Source: CAD feature listing. Evaluate the final solid. Frame: model axes, mm. Face numbers are marked on the shaded views. Give positions to 0.01 mm unless a question says otherwise; leave off trailing zeros. Loops run counter-clockwise (first coordinate to the right, second up) from the corner with the lowest first, then second, coordinate; pieces in that order, holes last. Notation, with made-up numbers: M -1.5,22 L 5.5,22 A13 ccw 5.5,31 Z; hole C 12,-29.5 d10. An arc over 180 degrees is marked long. Write item = value, one per line.
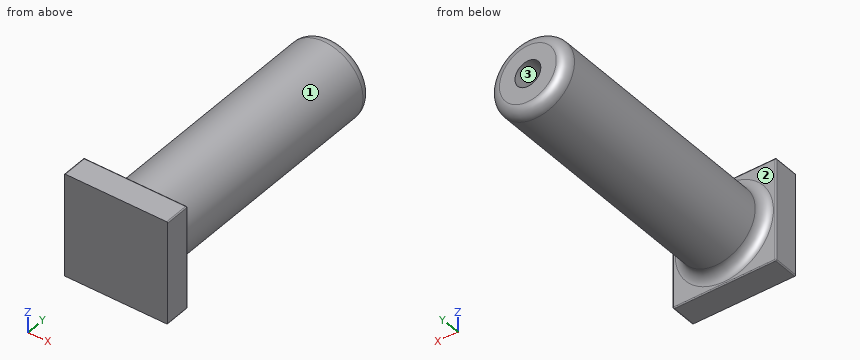
Autodesk Inventor part; units mm, degrees
ref_plane "YZ Plane" through (0, 0, 0) normal (1, 0, 0) x (0, 1, 0)
ref_plane "XZ Plane" through (0, 0, 0) normal (0, 1, 0) x (-1, 0, 0)
ref_plane "XY Plane" through (0, 0, 0) normal (0, 0, 1) x (1, 0, 0)
sketch "スケッチ1" plane through (0, 0, 0) normal (0, 1, 0) x (-1, 0, 0)
  line L0 (10, -10) -> (-10, -10)
  line L1 (-10, -10) -> (-10, 10)
  line L2 (-10, 10) -> (10, 10)
  line L3 (10, 10) -> (10, -10)
  line L4 (10, -10) -> (-10, 10) construction
  line L5 (-10, -10) -> (10, 10) construction
  point P0 (0, 0)
  dimension "d0" = 20
  dimension "d1" = 20
extrude "押し出し1" add sketch "スケッチ1" along normal blind 5
fillet "フィレット1" radius 0.2 8 edges at (0, 5, 10) (-10, 5, 0) (0, 5, -10) (10, 5, 0) (10, 2.5, 10) (-10, 2.5, 10) (-10, 2.5, -10) (10, 2.5, -10)
sketch "スケッチ2" plane through (0, 5, 0) normal (0, 1, 0) x (1, 0, 0)
  circle A0 centre (0, 0) radius 7.5
  circle A1 centre (0, 0) radius 2.5
  dimension "d9" = 2
  dimension "d5" = 15
  dimension "d6" = 5
extrude "押し出し2" add sketch "スケッチ2" along normal blind 50
fillet "フィレット2" radius 2 3 edges at (-7.5, 55, 0) (-7.5, 5, 0) (-2.5, 5, 0)
properties part number "baseA"
1. Cut plane A-A, the plane y = 42. Return the cut outline in (x, z).
Derived:
outline = C 0,0 d15; hole C 0,0 d5
2. Material intervals for probe 1 along X at (y, z) = (16, 0.25); probe 2 along Z at (x, y) = (0, 20); probe 3 along Y at (x, z) = (-6.25, -8.5), sorted ascending. Write a range as from..to.
Derived:
probe_1 = -7.5..-2.49, 2.49..7.5
probe_2 = -7.5..-2.5, 2.5..7.5
probe_3 = 0..5
3. First-contact query: pin 1 Ø1.5 at (y, z) = (41.5, 0) entering from -X; pin 2 Ø6 at (x, y) = (0.5, 10.5) entering from -Z; pin 3 Ø4 at (x, y) = (-7, 44.5) entering from +Z. Flat tips, straight axial feed; report the tip coordinate or a pass-through.
Derived:
pin_1 = -7.5
pin_2 = -7.5
pin_3 = 5.59
4. Pull-direction query (Z, two-part tool) for the marked faces 1, 2 and 3; classes: +Z half, -Z half, draft (parallel to the pull), parting line (faces both ways), or undercut.
Derived:
face_1 = parting line
face_2 = draft
face_3 = undercut
